Check sheet for the modelled part. Datum: model origin and axes. Units: mm. Face numbers are marked on the shaded views. A direction names the side the tool comes from. Give positions to 0.01 mm unless a question says otherwise; leave off trailing zeros. Order: outer loops, then holes, each group sorted by start corner. A loop starts at its lowest first (then second) coordinate and runs counter-clockwise, first axis right, second up.
from build123d import *

# Parameters (mm, degrees)
SKETCH1_W                 = 31.5
SKETCH1_H                 = 55
SKETCH1_W_2               = 5
SKETCH1_H_2               = 24
CHAMFER1_SIZE             = 5
CHAMFER1_SIZE2            = 7.140740034
CHAMFER2_SIZE             = 2
CHAMFER2_SIZE2            = 2.856296013
F_4_0MM_DOWEL_HOLE1_D     = 4
F_4_0MM_DOWEL_HOLE1_DEPTH = 20
F_4_0MM_DOWEL_HOLE1_TIP   = 1.201721238


with BuildPart() as part:
    # Sketch1 → Revolve1 (revolve)
    with BuildSketch(Plane.XY):
        with Locations((15.75, 27.5)):
            Rectangle(SKETCH1_W, SKETCH1_H)
        with Locations((2.5, 67)):
            Rectangle(SKETCH1_W_2, SKETCH1_H_2)
    revolve(axis=Axis((0, 55, 0), (0, 1, 0)))

    # Chamfer1
    chamfer1_edges = [part.edges().sort_by_distance(p)[0] for p in [
        (-31.5, 55, 0),
    ]]
    chamfer1_side = [part.faces().sort_by_distance(p)[0] for p in [
        (-30.609045456, 55, 0),
    ]]
    chamfer(chamfer1_edges, length=CHAMFER1_SIZE, length2=CHAMFER1_SIZE2, reference=chamfer1_side[0])

    # Chamfer2
    chamfer2_edges = [part.edges().sort_by_distance(p)[0] for p in [
        (-31.5, 0, 0),
    ]]
    chamfer2_side = [part.faces().sort_by_distance(p)[0] for p in [
        (-31.5, 23.929629983, 0),
    ]]
    chamfer(chamfer2_edges, length=CHAMFER2_SIZE, length2=CHAMFER2_SIZE2, reference=chamfer2_side[0])

    # Ø4.0mm Dowel Hole1
    with Locations(Plane(origin=(0, 55, 0), x_dir=(1, 0, 0), z_dir=(0, 1, 0))):
        with Locations((15, 0), (0, 22), (22, 0), (0, -22), (-22, 0), (0, 15), (-15, 0), (0, -15)):
            Hole(F_4_0MM_DOWEL_HOLE1_D / 2, depth=F_4_0MM_DOWEL_HOLE1_DEPTH)
            with Locations((0, 0, -(F_4_0MM_DOWEL_HOLE1_DEPTH + F_4_0MM_DOWEL_HOLE1_TIP / 2))):  # 118° drill point
                Cone(0, F_4_0MM_DOWEL_HOLE1_D / 2, F_4_0MM_DOWEL_HOLE1_TIP, mode=Mode.SUBTRACT)


solid = part.part
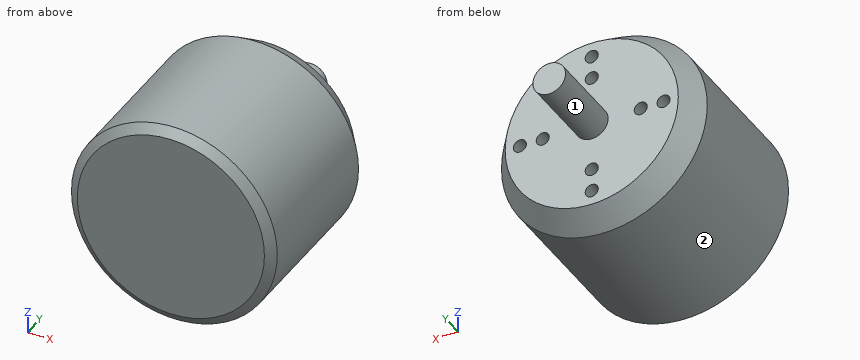
1) Material ranges on L1, parallel to Z at x = 0, y = 19; L2, parallel to X at y = 50, z = 15; L3, parallel to Y at x = 21, z = 14, recorded low to high.
Recorded:
L1: z = -31.5 to 31.5
L2: x = -25.98 to -2, 2 to 25.98
L3: y = 0 to 55
2) Set-up check for the marked faces 1 and 2: record each of +Z, -Z, +X, -X, +Y, -Y from which the full face is reachable in a straight line by a thin tool's end or side.
Recorded:
face 1: +Y
face 2: +Y, -Y
3) Section check A-A, the plane y = 50. State how many separate pieces and enclosed holes the cut face has, then the cut area to 3 significant figures.
Recorded:
separate pieces: 1
enclosed holes: 8
area: 2,730 mm2
4) Section check B-B, the plane y = 6.5. Record the cut outline in (x, z).
Recorded:
outline: circle Ø63 at (0, 0)
5) Depth check by flat-ended pin: pin 1 Ø5 at (x, z) = (0, -22) entering from +Y; pin 2 Ø2.5 at (x, z) = (0, -15) entering from +Y; pin 3 Ø6 at (x, y) = (-1, 53) entering from -Z. Enter the tip coordinate at first touch or a pass-through.
Recorded:
pin 1: stops at y = 55
pin 2: stops at y = 34.55
pin 3: stops at z = -29.99
